```python
from build123d import *

# Parameters (mm, degrees)
SKETCH1_W           = 40
SKETCH1_H           = 40
BOSS_EXTRUDE1_DEPTH = 40
CUT_EXTRUDE1_DEPTH  = 40
SKETCH3_W           = 20
SKETCH3_H           = 20
CUT_EXTRUDE2_DEPTH  = 40
SKETCH5_W           = 20
SKETCH5_H           = 20
CUT_EXTRUDE4_DEPTH  = 40
CUT_EXTRUDE5_DEPTH  = 40


with BuildPart() as part:
    # Sketch1 → Boss-Extrude1 (new body)
    with BuildSketch(Plane.XY):
        with Locations((20, 20)):
            Rectangle(SKETCH1_W, SKETCH1_H)
    extrude(amount=BOSS_EXTRUDE1_DEPTH)

    # Sketch2 → Cut-Extrude1 (cut)
    with BuildSketch(Plane.XY.offset(40)):
        Polygon((40, 40), (0, 20), (0, 40), align=None)
    extrude(amount=-CUT_EXTRUDE1_DEPTH, mode=Mode.SUBTRACT)

    # Sketch3 → Cut-Extrude2 (cut)
    with BuildSketch(Plane(origin=(40, 0, 0), x_dir=(0, 0, -1), z_dir=(1, 0, 0))):
        with Locations((-30, 30)):
            Rectangle(SKETCH3_W, SKETCH3_H)
    extrude(amount=-CUT_EXTRUDE2_DEPTH, mode=Mode.SUBTRACT)

    # Sketch5 → Cut-Extrude4 (cut)
    with BuildSketch(Plane(origin=(0, 20, 0), x_dir=(1, 0, 0), z_dir=(0, 1, 0))):
        with Locations((30, -30)):
            Rectangle(SKETCH5_W, SKETCH5_H)
    extrude(amount=-CUT_EXTRUDE4_DEPTH, mode=Mode.SUBTRACT)

    # Sketch6 → Cut-Extrude5 (cut)
    with BuildSketch(Plane.ZY):
        Polygon((0, 20), (20, 0), (0, 0), align=None)
    extrude(amount=-CUT_EXTRUDE5_DEPTH, mode=Mode.SUBTRACT)


solid = part.part
```
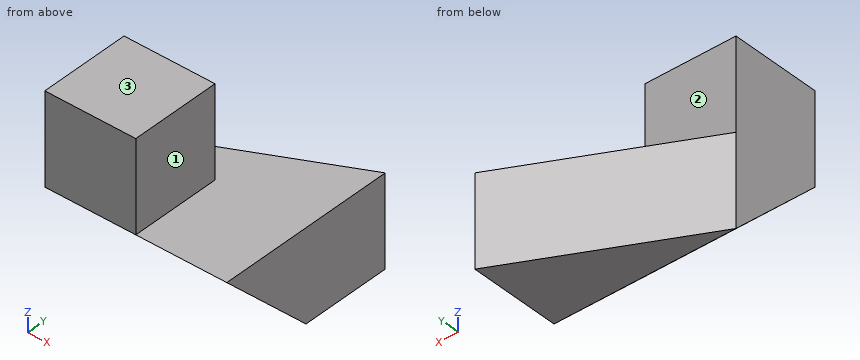
Model file for the job. Use its own axes, mm. Face numbers are marked on the shaded views. A direction names the side the tool comes from. Coordinates: 2 decimals unless noted, no trailing zeros. Loops run counter-clockwise (first coordinate to the right, second up) from the corner with the lowest first, then second, coordinate; pieces in that order, holes last. Notation, with made-up numbers: (-30, 10) -> (-19, 10) arc R25 cw to (-19, 43) -> close; hole circle Ø8 at (-14, 76.5). An arc over 180 degrees is marked (long way). Answer as a JSON object with one key per item and string values.
Q1. Cut at B-B (x = 19). List the corners of the cut face in (y, z), and give its area (3 significant figures).
Report:
{"outline": "(0, 20) -> (20, 0) -> (29.5, 0) -> (29.5, 20) -> (20, 20) -> (20, 40) -> (0, 40) -> close", "area": "790 mm2"}
Q2. Cut at D-D (y = 13.5). List the corners of the cut face in (x, z), and give its area (3 significant figures).
Report:
{"outline": "(0, 6.5) -> (40, 6.5) -> (40, 20) -> (20, 20) -> (20, 40) -> (0, 40) -> close", "area": "940 mm2"}
Q3. Probe probe 1 along Y at (x, z) = (2.5, 32.5). List the from-to ranges inside material, lowest first.
Report:
{"probe 1": "y = 0 to 20"}
Q4. Cut at C-C (z = 5). List the corners of the cut face in (x, y).
Report:
{"outline": "(0, 15) -> (40, 15) -> (40, 40) -> (0, 20) -> close"}
Q5. Flat gauge pins, fed straight in: P1, Ø10, axis at x = 9, z = 30, coming from the +Y side; P2, Ø2, axis at x = 11.5, z = 7.5, coming from the +Y side; P3, Ø10, axis at x = 7.5, y = 26, coming from the +Z side. Where does each tip first touch, or does it go through?
Report:
{"P1": "stops at y = 20", "P2": "stops at y = 26.25", "P3": "stops at z = 20"}
Q6. Cut at A-A (y = 18). List the corners of the cut face in (x, z).
Report:
{"outline": "(0, 2) -> (40, 2) -> (40, 20) -> (20, 20) -> (20, 40) -> (0, 40) -> close"}
Q7. 3-axis set-ups, long thin cutter, end or side, ignore diameter. For the marked faces 1, 2 and 3: which of +Z, -Z, +X, -X, +Y, -Y reach the whole face in a straight line?
Report:
{"face 1": "+Z, +X, +Y, -Y", "face 2": "+Z, +X, -X, +Y", "face 3": "+Z, +X, -X, +Y, -Y"}
